Check sheet for the modelled part. Datum: model origin and axes. Units: mm. A direction names the side the tool comes from. Round coordinates to 2 decimals unless told otherwise and drop trailing zeros. Write each loop counter-clockwise with the first axis right and the second up, starting at its lowest first coordinate (ties: lowest second). Pieces come first, ordered by that corner, then holes. Notation, with made-up numbers: (19, 5.25) -> (47, 5.25) arc R27 cw to (47, 38.25) -> close; hole circle Ø1 at (-28, 78.5). An arc over 180 degrees is marked (long way). Answer as a JSON object with one key per item and string values. Group by question number.
```python
from build123d import *

# Parameters (mm, degrees)
F0_W      = 324.4502871967
F0_H      = 65
F1_DEPTH  = 50
F2_R      = 49.99999
F3_W      = 60
F3_H      = 50
F4_DEPTH  = 25
F6_DEPTH  = 65
F8_DEPTH  = 65
F9_W      = 10
F9_H      = 50
F10_DEPTH = 25


# Not quite as in the source:
# - a fillet or chamfer is up to 0.001 mm smaller than in the source, because OpenCascade refuses the exact size


with BuildPart() as f1:
    # F0 (on Top) → F1 (new body)
    with BuildSketch(Plane.XY):
        with Locations((69.7921998799, -49.3180742487)):
            Rectangle(F0_W, F0_H)
    extrude(amount=F1_DEPTH)

    # F2 (radius 50 in the source; OpenCascade refuses exactly that, so slightly less here)
    f2_edges = [f1.edges().sort_by_distance(p)[0] for p in [
        (232.017343, -49.318074, 50),
    ]]
    fillet(f2_edges, radius=F2_R)

    # F3 (on face) → F4 (cut)
    with BuildSketch(Plane.XY.offset(50)):
        with Locations((-50.6331702159, -48.4395725653)):
            Rectangle(F3_W, F3_H)
        with Locations((26.5513133067, -48.4395725653)):
            Rectangle(F3_W, F3_H)
        with Locations((117.3280163615, -48.4395725653)):
            Rectangle(F3_W, F3_H)
    extrude(amount=-F4_DEPTH, mode=Mode.SUBTRACT)

    # F5 (on face) → F6 (cut)
    with BuildSketch(Plane.XZ.offset(81.8180742487)):
        with BuildLine():
            ThreePointArc((211.8422013521, 0), (204.3422013521, 7.5), (196.8422013521, 0))
            Line((196.8422013521, 0), (211.8422013521, 0))
        make_face()
        with BuildLine():
            ThreePointArc((165.3422039747, 0), (157.8422039747, 7.5), (150.3422039747, 0))
            Line((150.3422039747, 0), (165.3422039747, 0))
        make_face()
        with BuildLine():
            ThreePointArc((-22.1578053385, 0), (-29.6578053385, 7.5), (-37.1578053385, 0))
            Line((-37.1578053385, 0), (-22.1578053385, 0))
        make_face()
        with BuildLine():
            Line((-85.1578038931, 0), (-70.1578038931, 0))
            ThreePointArc((-70.1578038931, 0), (-77.6578038931, 7.5), (-85.1578038931, 0))
        make_face()
    extrude(amount=F6_DEPTH, mode=Mode.SUBTRACT)

    # F7 (on face) → F8 (join)
    with BuildSketch(Plane(origin=(0, -16.8180742487, 0), x_dir=(-1, 0, 0), z_dir=(0, 1, 0))):
        with BuildLine():
            Line((-213.942207098, 0), (-198.942207098, 0))
            ThreePointArc((-198.942207098, 0), (-206.442207098, 7.5), (-213.942207098, 0))
        make_face()
        with BuildLine():
            ThreePointArc((-213.942207098, 0), (-206.442207098, -7.5), (-198.942207098, 0))
            Line((-198.942207098, 0), (-213.942207098, 0))
        make_face()
        with BuildLine():
            Line((-159.0422022343, 0), (-174.0422022343, 0))
            ThreePointArc((-174.0422022343, 0), (-166.5422022343, -7.5), (-159.0422022343, 0))
        make_face()
        with BuildLine():
            ThreePointArc((-159.0422022343, 0), (-166.5422022343, 7.5), (-174.0422022343, 0))
            Line((-174.0422022343, 0), (-159.0422022343, 0))
        make_face()
        with BuildLine():
            Line((-62.2921998799, 0), (-77.2921998799, 0))
            ThreePointArc((-77.2921998799, 0), (-69.7921998799, -7.5), (-62.2921998799, 0))
        make_face()
        with BuildLine():
            ThreePointArc((-62.2921998799, 0), (-69.7921998799, 7.5), (-77.2921998799, 0))
            Line((-77.2921998799, 0), (-62.2921998799, 0))
        make_face()
        with BuildLine():
            Line((46.7355581226, 0), (30.5800629554, 0))
            ThreePointArc((30.5800629554, 0), (38.657810539, -8.0777475836), (46.7355581226, 0))
        make_face()
        with BuildLine():
            ThreePointArc((62.9578086734, 0), (70.4578086734, -7.5), (77.9578086734, 0))
            Line((77.9578086734, 0), (62.9578086734, 0))
        make_face()
    extrude(amount=-F8_DEPTH)

    # F9 (on face) → F10 (join)
    with BuildSketch(Plane.XY.offset(50)):
        with Locations((-85.6331702159, -48.4395725653)):
            Rectangle(F9_W, F9_H)
        with Locations((-8.4486866933, -48.4395725653)):
            Rectangle(F9_W, F9_H)
        with Locations((82.3280163615, -48.4395725653)):
            Rectangle(F9_W, F9_H)
    extrude(amount=F10_DEPTH)


solid = f1.part
```
(1) Section check B-B on x = -55. Record the cut outline in (y, z), then the cut area to 3 significant figures.
(2) Access from +Z, -Z, +X, -X, +Y, -Y to the whole of each face (thin tool, end or side, straight path). Record for faces 1 (the flat face through (-85, -49, 0)), 2 (the flat face through (-13.449, -49, 62)), 3 (the flat face through (-51, -23.44, 38)).
(3) Scan lines: line 1 along X through (y, z) = (-64, 62.5); line 2 along X through (y, z) = (-55, 26); line 3 along X through (y, z) = (-52, 34). Record each from-to range of solid material in increasing order.
(4) Section check D-D on z = 38. Record the cut outline in (x, y).
(5) Go/stop test with flat-tipped pins: pin 1 Ø5 at (x, z) = (81.5, 60.5) entering from +Y; pin 2 Ø10 at (y, z) = (-71.5, 61) entering from +X; pin 3 Ø12 at (x, y) = (-55, -43.5) entering from -Z. Record where each tip stops, or that it passes through.
(6) Section check A-A on z = 60. Record the cut outline in (x, y), then the cut area to 3 significant figures.
(7) Release check for a two-part mould opening along X. For faces 4 (the cylindrical face through (206.6, -48.9, -7.5)), 5 (the flat face through (-9, -73.44, 62)) record: pulls with the +X half, pulls with the -X half, needs draft (parallel to the pull), parting line crosses it, or undercut.
Data:
{
 "1": {"outline": "(-81.82, 0) -> (-16.82, 0) -> (-16.82, 50) -> (-23.44, 50) -> (-23.44, 25) -> (-73.44, 25) -> (-73.44, 50) -> (-81.82, 50) -> close", "area": "2,000 mm²"},
 "2": {"face 1": "-Z, -X, +Y, -Y", "face 2": "+Z, +Y, -Y", "face 3": "+Z"},
 "3": {"line 1": "x = -90.63 to -80.63, -13.45 to -3.45, 77.33 to 87.33", "line 2": "x = -92.43 to -80.63, -20.63 to -3.45, 56.55 to 87.33, 147.33 to 224.73", "line 3": "x = -92.43 to -80.63, -20.63 to -3.45, 56.55 to 87.33, 147.33 to 218.68"},
 "4": {"outline": "(-92.43, -81.82) -> (214.51, -81.82) -> (214.51, -16.82) -> (-92.43, -16.82) -> close; hole (-80.63, -73.44) -> (-20.63, -73.44) -> (-20.63, -23.44) -> (-80.63, -23.44) -> close; hole (-3.45, -73.44) -> (56.55, -73.44) -> (56.55, -23.44) -> (-3.45, -23.44) -> close; hole (87.33, -73.44) -> (147.33, -73.44) -> (147.33, -23.44) -> (87.33, -23.44) -> close"},
 "5": {"pin 1": "stops at y = -23.44", "pin 2": "stops at x = 87.33", "pin 3": "stops at z = 0"},
 "6": {"outline": "(-90.63, -73.44) -> (-80.63, -73.44) -> (-80.63, -23.44) -> (-90.63, -23.44) -> close; (-13.45, -73.44) -> (-3.45, -73.44) -> (-3.45, -23.44) -> (-13.45, -23.44) -> close; (77.33, -73.44) -> (87.33, -73.44) -> (87.33, -23.44) -> (77.33, -23.44) -> close", "area": "1,500 mm²"},
 "7": {"face 4": "undercut", "face 5": "needs draft"}
}
